Check sheet for the modelled part. Datum: model origin and axes. Units: mm. A direction names the side the tool comes from. Coordinates: 2 decimals unless noted, no trailing zeros. Loops run counter-clockwise (first coordinate to the right, second up) from the corner with the lowest first, then second, coordinate; pieces in that order, holes last. Notation, with made-up numbers: M -7,44 L 4,44 A28 cw 4,70 Z; hole C 11,46.5 d2. An arc over 180 degrees is marked long. Answer in a Markdown table with one row per item. Add a question column.
```python
from build123d import *

# Parameters (mm, degrees)
SKETCH_1_R          = 1.55
EXTRUDE_1_DEPTH     = 5
SKETCH_2_R          = 1.1
CUT_EXTRUDE_1_DEPTH = 5


with BuildPart() as part:
    # 草图1 → 凸台-拉伸1 (new body)
    with BuildSketch(Plane(origin=(0, 0, 0), x_dir=(0, 0, -1), z_dir=(1, 0, 0))):
        Polygon((-4, 10.2), (-4, -3.2), (15, -3.2), (15, -0.2), (4, -0.2), (4, 10.2), align=None)
        Circle(SKETCH_1_R, mode=Mode.SUBTRACT)
        with Locations((0, 7)):
            Circle(SKETCH_1_R, mode=Mode.SUBTRACT)
    extrude(amount=EXTRUDE_1_DEPTH)

    # 草图2 → 切除-拉伸1 (cut)
    with BuildSketch(Plane(origin=(0, -0.2, 0), x_dir=(1, 0, 0), z_dir=(0, 1, 0))):
        with Locations(Location((2.5, 7, 0), (0, 0, 270))):
            Circle(SKETCH_2_R)
        with Locations(Location((2.5, 12, 0), (0, 0, 270))):
            Circle(SKETCH_2_R)
    extrude(amount=-CUT_EXTRUDE_1_DEPTH, mode=Mode.SUBTRACT)


solid = part.part
```
Q1. Cross-section at D-D (x = 0.85). Record the cut outline in (y, z), plus the area to 3 significant figures.
Q2. Go/stop test with flat-tipped pins: pin 1 (1.5 mm diameter, centred on x = 1.5, y = 3, fed in from -Z); pin 2 (1.5 mm diameter, centred on x = 1.5, z = -10.5, fed in from +Y). Record where each tip stops, or that it passes through.
Q3. Cross-section at A-A (z = 0). Record the cut outline in (x, y).
Q4. Access from +Z, -Z, +X, -X, +Y, -Y to the whole of each face (thin tool, end or side, straight path). Record for faces 4 (the face through (2, 5, -4)), 5 (the face through (2, 10.2, 0)).
Q5. Thickness scan on L1, parallel to X at y = -1.4, z = -7; L2, parallel to Y at x = 2.15, z = 0; L3, parallel to Z at x = 3.2, y = 9.75. Record the ranges inside material, lowest first.
Q6. Cross-section at B-B (y = -1). Record the cut outline in (x, z).
Q7. Mould release check, pull along Z, two halves, no side actions. Record for faces 1 (the face through (2.465, -1.375, -0.715)), 2 (the face through (2, 4, 4)), 3 (the face through (2, -0.2, -10)): released by +Z, released by -Z, zero draft, split by the parting line, or undercut.
Q8. Cross-section at C-C (z = -7). Record the cut outline in (x, y), plus the area to 3 significant figures.
Answer key:
| question | item | result |
|---|---|---|
| 1 | outline | M -3.2,-15 L -0.2,-15 L -0.2,-4 L 10.2,-4 L 10.2,4 L -3.2,4 Z; hole C 0,0 d3.1; hole C 7,0 d3.1 |
| 1 | area | 125 mm^2 |
| 2 | pin 1 | z = -4 |
| 2 | pin 2 | y = -0.2 |
| 3 | outline | M 0,-3.2 L 5,-3.2 L 5,-1.55 L 0,-1.55 Z; M 0,1.55 L 5,1.55 L 5,5.45 L 0,5.45 Z; M 0,8.55 L 5,8.55 L 5,10.2 L 0,10.2 Z |
| 4 | face 4 | -Z, +X, -X, +Y |
| 4 | face 5 | +Z, -Z, +X, -X, +Y |
| 5 | L1 | 0 to 1.4, 3.6 to 5 |
| 5 | L2 | -3.2 to -1.55, 1.55 to 5.45, 8.55 to 10.2 |
| 5 | L3 | -4 to 4 |
| 6 | outline | M 0,-15 L 5,-15 L 5,-1.18 L 0,-1.18 Z; M 0,1.18 L 5,1.18 L 5,4 L 0,4 Z; hole C 2.5,-12 d2.2; hole C 2.5,-7 d2.2 |
| 7 | face 1 | undercut |
| 7 | face 2 | released by +Z |
| 7 | face 3 | zero draft |
| 8 | outline | M 0,-3.2 L 1.4,-3.2 L 1.4,-0.2 L 0,-0.2 Z; M 3.6,-3.2 L 5,-3.2 L 5,-0.2 L 3.6,-0.2 Z |
| 8 | area | 8.40 mm^2 |
